```python
from build123d import *

# Parameters (mm, degrees)
F0_W     = 100
F0_H     = 194
F0_R     = 4.25
F0_R_2   = 2.5
F0_R_3   = 5
F0_R_4   = 23.5
F1_DEPTH = 12
F2_SIZE  = 0.5
F3_R     = 3.25
F4_DEPTH = 25
F5_SIZE  = 0.5


with BuildPart() as f1:
    # F0 (on Top) → F1 (new body)
    with BuildSketch(Plane.XY):
        with Locations((0, 31)):
            Rectangle(F0_W, F0_H)
        with Locations((-40, -57)):
            Circle(F0_R, mode=Mode.SUBTRACT)
        with Locations((-29, 0)):
            Circle(F0_R_2, mode=Mode.SUBTRACT)
        with Locations((0, -57)):
            Circle(F0_R_3, mode=Mode.SUBTRACT)
        with Locations((0, -29)):
            Circle(F0_R_2, mode=Mode.SUBTRACT)
        with Locations((40, -57)):
            Circle(F0_R, mode=Mode.SUBTRACT)
        Circle(F0_R_4, mode=Mode.SUBTRACT)
        with Locations((0, 29)):
            Circle(F0_R_2, mode=Mode.SUBTRACT)
        with Locations((29, 0)):
            Circle(F0_R_2, mode=Mode.SUBTRACT)
        with Locations((-40, 119)):
            Circle(F0_R, mode=Mode.SUBTRACT)
        with Locations((0, 119)):
            Circle(F0_R_3, mode=Mode.SUBTRACT)
        with Locations((40, 119)):
            Circle(F0_R, mode=Mode.SUBTRACT)
    extrude(amount=F1_DEPTH)

    # F2
    f2_edges = [f1.edges().sort_by_distance(p)[0] for p in [
        (-35.75, 119, 6),
        (-44.25, 119, 0),
        (-44.25, 119, 12),
        (5, 119, 6),
        (-5, 119, 0),
        (-5, 119, 12),
        (44.25, 119, 6),
        (35.75, 119, 0),
        (35.75, 119, 12),
        (23.5, 0, 6),
        (-23.5, 0, 0),
        (-23.5, 0, 12),
        (-35.75, -57, 6),
        (-44.25, -57, 0),
        (-44.25, -57, 12),
        (5, -57, 6),
        (-5, -57, 0),
        (-5, -57, 12),
        (44.25, -57, 6),
        (35.75, -57, 0),
        (35.75, -57, 12),
        (2.5, 29, 6),
        (-2.5, 29, 0),
        (-2.5, 29, 12),
        (-26.5, 0, 6),
        (-31.5, 0, 0),
        (-31.5, 0, 12),
        (2.5, -29, 6),
        (-2.5, -29, 0),
        (-2.5, -29, 12),
        (31.5, 0, 6),
        (26.5, 0, 0),
        (26.5, 0, 12),
    ]]
    chamfer(f2_edges, length=F2_SIZE)

    # F3 (on face) → F4 (cut)
    with BuildSketch(Plane.XY.offset(12)):
        with Locations((-41, 31)):
            Circle(F3_R)
        with Locations((41, 31)):
            Circle(F3_R)
        with Locations((41, 101)):
            Circle(F3_R)
        with Locations((-41, 101)):
            Circle(F3_R)
        with Locations((41, -39)):
            Circle(F3_R)
        with Locations((-41, -39)):
            Circle(F3_R)
    extrude(amount=-F4_DEPTH, mode=Mode.SUBTRACT)

    # F5
    f5_edges = [f1.edges().sort_by_distance(p)[0] for p in [
        (-44.25, 101, 12),
        (-37.75, 101, 6),
        (-44.25, 101, 0),
        (37.75, 101, 12),
        (44.25, 101, 6),
        (37.75, 101, 0),
        (37.75, 31, 12),
        (44.25, 31, 6),
        (37.75, 31, 0),
        (-44.25, 31, 12),
        (-37.75, 31, 6),
        (-44.25, 31, 0),
        (-44.25, -39, 12),
        (-37.75, -39, 6),
        (-44.25, -39, 0),
        (37.75, -39, 12),
        (44.25, -39, 6),
        (37.75, -39, 0),
    ]]
    chamfer(f5_edges, length=F5_SIZE)


solid = f1.part
```
Could you check a few things on this model? Use its own coordinates, in mm. Round coordinates to 2 decimals unless told otherwise and drop trailing zeros. Loops run counter-clockwise (first coordinate to the right, second up) from the corner with the lowest first, then second, coordinate; pieces in that order, holes last. Notation, with made-up numbers: (36, 88) - (73, 88) arc R25 cw to (73, 107) - close; hole circle Ø5 at (78.5, -25). An arc over 180 degrees is marked (long way). Answer as CSV lines item,"result".
1. I want a section at B-B on x = 29. List the corners of the cut face in (y, z) for me, then the cut area to 3 significant figures.
Filled in:
outline,"(-66, 0) - (-3, 0) - (-2.5, 0.5) - (-2.5, 11.5) - (-3, 12) - (-66, 12) - close; (2.5, 0.5) - (3, 0) - (128, 0) - (128, 12) - (3, 12) - (2.5, 11.5) - close"
area,"2,270 mm^2"
2. Please list where these lines run through material, in increasing order: line 1 along Y through (x, z) = (41, 3.25); line 2 along Y through (x, z) = (40, 6); line 3 along X through (y, z) = (120.5, 8.75). Write a range as [from, to].
Filled in:
line 1,"y = [-66, -61.13], [-52.87, -42.25], [-35.75, 27.75], [34.25, 97.75], [104.25, 114.87], [123.13, 128]"
line 2,"y = [-66, -61.25], [-52.75, -42.09], [-35.91, 27.91], [34.09, 97.91], [104.09, 114.75], [123.25, 128]"
line 3,"x = [-50, -43.98], [-36.02, -4.77], [4.77, 36.02], [43.98, 50]"
3. I want a section at D-D on y = -39. List the corners of the cut face in (x, z) for me, then the cut area to 3 significant figures.
Filled in:
outline,"(-50, 0) - (-44.75, 0) - (-44.25, 0.5) - (-44.25, 11.5) - (-44.75, 12) - (-50, 12) - close; (-37.75, 0.5) - (-37.25, 0) - (37.25, 0) - (37.75, 0.5) - (37.75, 11.5) - (37.25, 12) - (-37.25, 12) - (-37.75, 11.5) - close; (44.25, 0.5) - (44.75, 0) - (50, 0) - (50, 12) - (44.75, 12) - (44.25, 11.5) - close"
area,"1,040 mm^2"
4. We'd pull the mould along X, two halves only. Please class faces 1 (the face through (-1, 32, 12)), 2 (the face through (-1.08, 114.12, 5.92)): +X half, -X half, draft (parallel to the pull), parting line (faces both ways), or undercut.
Filled in:
face 1,"draft"
face 2,"undercut"
5. I want a section at C-C on z = 9.5. Count the separate pieces of the cut face and the enclosed holes in it, then the cut area to 3 significant figures.
Filled in:
separate pieces,"1"
enclosed holes,"17"
area,"17,000 mm^2"
6. I want a section at A-A on y = 119. List the corners of the cut face in (x, z) for me.
Filled in:
outline,"(-50, 0) - (-44.75, 0) - (-44.25, 0.5) - (-44.25, 11.5) - (-44.75, 12) - (-50, 12) - close; (-35.75, 0.5) - (-35.25, 0) - (-5.5, 0) - (-5, 0.5) - (-5, 11.5) - (-5.5, 12) - (-35.25, 12) - (-35.75, 11.5) - close; (5, 0.5) - (5.5, 0) - (35.25, 0) - (35.75, 0.5) - (35.75, 11.5) - (35.25, 12) - (5.5, 12) - (5, 11.5) - close; (44.25, 0.5) - (44.75, 0) - (50, 0) - (50, 12) - (44.75, 12) - (44.25, 11.5) - close"
7. For pin 1 Ø7 at (x, y) = (-40, -57) entering from -Z, with a flat end and sliding along its axis, tell me the tip position at first contact or that it passes through.
Filled in:
pin 1,"passes through"
